from build123d import *

# Parameters (mm, degrees)
F1_DEPTH = 50
F3_START = -144.7303891182
F2_R     = 17.5
F3_DEPTH = 29.2989462614
F4_R     = 5
F6_D     = 25
F7_R     = 5


with BuildPart() as f1:
    # F0 (on Top) → F1 (new body)
    with BuildSketch(Plane.XY):
        with BuildLine():
            ThreePointArc((-57.8447732054, 127.4911064067), (0, 140), (57.8447732054, 127.4911064067))
            Line((57.8447732054, 127.4911064067), (60, 127.4911064067))
            Line((60, 127.4911064067), (60, 137.4772708487))
            ThreePointArc((60, 137.4772708487), (0, 150), (-60, 137.4772708487))
            Line((-60, 137.4772708487), (-60, 127.4911064067))
            Line((-60, 127.4911064067), (-57.8447732054, 127.4911064067))
        make_face()
    extrude(amount=F1_DEPTH)

    # F2 (on Front) → F3 (join)
    with BuildSketch(Plane.XZ.offset(F3_START)):
        with Locations((0, 25)):
            Circle(F2_R)
    extrude(amount=-F3_DEPTH)

    # F4
    f4_edges = [f1.edges().sort_by_distance(p)[0] for p in [
        (-17.5, 148.975669, 25),
    ]]
    fillet(f4_edges, radius=F4_R)

    # F6 (through all)
    with Locations(Plane(origin=(0, 174.0293353796, 0), x_dir=(-1, 0, 0), z_dir=(0, 1, 0))):
        with Locations((0, 25)):
            Hole(F6_D / 2)

    # F7
    f7_edges = [f1.edges().sort_by_distance(p)[0] for p in [
        (-60, 132.484189, 50),
        (-60, 137.477271, 25),
        (-60, 132.484189, 0),
        (60, 132.484189, 50),
        (60, 137.477271, 25),
        (60, 132.484189, 0),
    ]]
    fillet(f7_edges, radius=F7_R)


solid = f1.part
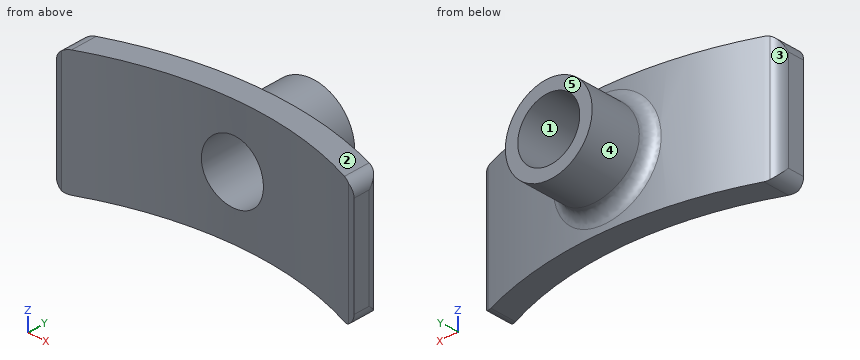
Input: part model. Units: mm. Frame: model coordinates. Face numbers are marked on the shaded views. A direction names the side the tool comes from. Coordinates: 2 decimals unless noted, no trailing zeros. Write each loop counter-clockwise with the first axis right and the second up, starting at its lowest first coordinate (ties: lowest second). Pieces come first, ordered by that corner, then holes. Notation, with made-up numbers: M -26,58.25 L 22,58.25 A16 ccw 22,68.25 Z; hole C -1.75,80.25 d9. An arc over 180 degrees is marked long. Answer as a JSON object with one key per item and string values. Group by question number.
(1) Mould query, pull axis Z, two halves, no side actions, for the marked faces 1, 2 and 3. Classes: pulls with the +Z half, pulls with the -Z half, needs draft (parallel to the pull), parting line crosses it, or undercut.
(2) Section C-C on y = 146.5. Output: boundary loops of the cut face in (x, z).
(3) Contact query for flat-ended pins moving along their axis: P1, Ø6, axis at y = 152.5, z = 36.5, coming from the +X side; P2, Ø8, axis at x = 43, y = 133.5, coming from the -Z side; P3, Ø10, axis at x = -40.5, z = 23.5, coming from the -Y side; P4, Ø2, axis at x = -5.5, y = 157.5, coming from the -Z side. Output: stop coordinate, or through.
(4) Section A-A on y = 160.5. Output: boundary loops of the cut face in (x, z).
(5) Set-up query: the marked faces 4 and 5. Return all of +Z, -Z, +X, -X, +Y, -Y with unobstructed straight access to the full face (end or side cutting, diameter ignored); none if empty.
(6) Section B-B on x = -43. Output: boundary loops of the cut face in (y, z).
(7) Ray query, line 1 along X through (y, z) = (158.5, 25); line 2 along Z through (x, y) = (0, 159); line 3 along Z through (x, y) = (9, 160.5). Return the intervals inside material, ascending. Write a range as [from, to].
Result set:
{
 "1": {"face 1": "undercut", "face 2": "pulls with the +Z half", "face 3": "needs draft"},
 "2": {"outline": "M -32.21,0 L 32.21,0 L 32.21,50 L -32.21,50 Z; hole C 0,25 d25"},
 "3": {"P1": "stops at x = 16.68", "P2": "stops at z = 0", "P3": "stops at y = 132.4", "P4": "stops at z = 8.09"},
 "4": {"outline": "C 0,25 d35; hole C 0,25 d25"},
 "5": {"face 4": "+Y", "face 5": "+Z, -Z, +X, -X, +Y"},
 "6": {"outline": "M 133.23,0 L 143.7,0 L 143.7,50 L 133.23,50 Z"},
 "7": {"line 1": "x = [-17.5, -12.5], [12.5, 17.5]", "line 2": "z = [7.5, 12.5], [37.5, 42.5]", "line 3": "z = [9.99, 16.33], [33.67, 40.01]"}
}
